Verification items for the finished model (mm, model axes). A direction names the side the tool comes from. Round coordinates to 2 decimals unless told otherwise and drop trailing zeros. Loops run counter-clockwise (first coordinate to the right, second up) from the corner with the lowest first, then second, coordinate; pieces in that order, holes last. Notation, with made-up numbers: (-39, -12.75) -> (18, -12.75) arc R36 ccw to (18, 22.25) -> close; hole circle Ø2 at (-15.75, 26). An arc over 180 degrees is marked (long way). Write item = value, one per line. Start each with the question number.
```python
from build123d import *

# Parameters (mm, degrees)
SALIENTE_EXTRUIR1_DEPTH = 8
REDONDEO1_R             = 0.01
CROQUIS3_R              = 2
CORTAR_EXTRUIR1_DEPTH   = 6
CROQUIS4_R              = 1.25
CORTAR_EXTRUIR2_DEPTH   = 10


with BuildPart() as part:
    # Croquis2 → Saliente-Extruir1 (new body)
    with BuildSketch(Plane(origin=(0, 0, 0), x_dir=(1, 0, 0), z_dir=(0, 1, 0))):
        with BuildLine():
            Line((-5, 40), (5, 40))
            ThreePointArc((5, 40), (19.142135624, 34.142135624), (25, 20))
            Line((25, 20), (25, -20))
            ThreePointArc((25, -20), (19.142135624, -34.142135624), (5, -40))
            Line((5, -40), (-5, -40))
            ThreePointArc((-5, -40), (-19.142135624, -34.142135624), (-25, -20))
            Line((-25, -20), (-25, 20))
            ThreePointArc((-25, 20), (-19.142135624, 34.142135624), (-5, 40))
        make_face()
    extrude(amount=SALIENTE_EXTRUIR1_DEPTH)

    # Redondeo1
    redondeo1_edges = [part.edges().sort_by_distance(p)[0] for p in [
        (-19.142135624, 8, 34.142135624),
        (0, 8, 40),
        (19.142135624, 8, 34.142135624),
        (25, 8, 0),
        (19.142135624, 8, -34.142135624),
        (0, 8, -40),
        (-19.142135624, 8, -34.142135624),
        (-25, 8, 0),
    ]]
    fillet(redondeo1_edges, radius=REDONDEO1_R)

    # Croquis3 → Cortar-Extruir1 (cut)
    with BuildSketch(Plane(origin=(0, 8, 0), x_dir=(1, 0, 0), z_dir=(0, 1, 0))):
        with Locations((-17, 0)):
            Circle(CROQUIS3_R)
    extrude(amount=-CORTAR_EXTRUIR1_DEPTH, mode=Mode.SUBTRACT)

    # Croquis4 → Cortar-Extruir2 (cut)
    with BuildSketch(Plane(origin=(0, 8, 0), x_dir=(1, 0, 0), z_dir=(0, 1, 0))):
        with Locations((-17, 0)):
            Circle(CROQUIS4_R)
    extrude(amount=-CORTAR_EXTRUIR2_DEPTH, mode=Mode.SUBTRACT)


solid = part.part
```
(1) Draft check along X on faces 1 (the cylindrical face through (19.297, 3.939, 33.986)), 2 (the flat face through (0, 4, 40)), 3 (the cylindrical face through (-15.845, 1.014, 0.479)). Enter one of: +X half, -X half, draft (parallel to the pull), parting line (faces both ways), or undercut.
(2) Depth check by flat-ended pin: pin 1 Ø2 at (x, y) = (8, 2) entering from -Z; pin 2 Ø1.2 at (x, z) = (-16.5, -1) entering from +Y; pin 3 Ø2 at (x, z) = (-17, 0) entering from +Y; pin 4 Ø4 at (x, z) = (6.5, 6) entering from -Y. Enter the tip coordinate at first touch or a pass-through.
(3) Section check A-A on y = 3.25. Enter the section's corners in (x, z), then the cut area to 3 significant figures.
(4) Access from +Z, -Z, +X, -X, +Y, -Y to the whole of each face (thin tool, end or side, straight path). Record for faces 4 (the flat face through (25, 4, 0)), 5 (the cylindrical face through (-18.6, 5, 1.2)).
(5) Scan lines: line 1 (Z direction, x = -17, y = 5.15); line 2 (X direction, y = 5.55, z = 0); line 3 (Z direction, x = -17, y = 0.9). Record each from-to range of solid material in increasing order. Write a range as [from, to].
Computed values:
q1.face_1 = +X half
q1.face_2 = draft
q1.face_3 = undercut
q2.pin_1 = -39.9
q2.pin_2 = 2
q2.pin_3 = through
q2.pin_4 = 0
q3.outline = (-25, -20) arc R20 ccw to (-5, -40) -> (5, -40) arc R20 ccw to (25, -20) -> (25, 20) arc R20 ccw to (5, 40) -> (-5, 40) arc R20 ccw to (-25, 20) -> close; hole circle Ø4 at (-17, 0)
q3.area = 3,640 mm²
q4.face_4 = +Z, -Z, +X, +Y, -Y
q4.face_5 = +Y
q5.line_1 = [-36, -2], [2, 36]
q5.line_2 = [-25, -19], [-15, 25]
q5.line_3 = [-36, -1.25], [1.25, 36]
